Could you check a few things on this model? Use its own coordinates, in mm. Face numbers are marked on the shaded views. A direction names the side the tool comes from. Round coordinates to 2 decimals unless told otherwise and drop trailing zeros. Loops run counter-clockwise (first coordinate to the right, second up) from the corner with the lowest first, then second, coordinate; pieces in that order, holes last. Notation, with made-up numbers: (78, 12.5) -> (129, 12.5) arc R22 cw to (129, 36.5) -> close; hole circle Ø6 at (71.25, -0.5). An arc over 180 degrees is marked (long way). One line per item, written item: value.
Autodesk Inventor part; units mm, degrees
ref_plane "YZ Plane" through (0, 0, 0) normal (1, 0, 0) x (0, 1, 0)
ref_plane "XZ Plane" through (0, 0, 0) normal (0, 1, 0) x (-1, 0, 0)
ref_plane "XY Plane" through (0, 0, 0) normal (0, 0, 1) x (1, 0, 0)
sketch "Sketch1" plane through (0, 0, 0) normal (0, 0, 1) x (1, 0, 0)
  circle A0 centre (0, 0) radius 9.5
  arc A1 (2, 11.5) -> (-2, 11.5) centre (0, 11.5) ccw
  line L0 (-2, 11.5) -> (-2, 9.2871)
  line L1 (2, 11.5) -> (2, 9.2871)
  line L2 (11.5, -2) -> (9.2871, -2)
  arc A2 (11.5, -2) -> (11.5, 2) centre (11.5, 0) ccw
  line L3 (11.5, 2) -> (9.2871, 2)
  line L4 (-2, -11.5) -> (-2, -9.2871)
  arc A3 (-2, -11.5) -> (2, -11.5) centre (0, -11.5) ccw
  line L5 (2, -11.5) -> (2, -9.2871)
  line L6 (-11.5, 2) -> (-9.2871, 2)
  arc A4 (-11.5, 2) -> (-11.5, -2) centre (-11.5, 0) ccw
  line L7 (-11.5, -2) -> (-9.2871, -2)
  line L8 (0, 0) -> (6.7175, 6.7175) construction
  line L9 (0, 0) -> (9.5, 0) construction
  line L10 (5.7012, 8.8174) -> (4.9765, 8.0923)
  line L11 (8.8174, 5.7012) -> (8.0925, 4.9761)
  arc A5 (8.8174, 5.7012) -> (5.7012, 8.8174) centre (0, 0) ccw
  arc A6 (-10.3078, 2) -> (-10.3696, 1.6499) centre (0, 0) ccw
  arc A7 (-10.3696, -1.6499) -> (-10.3078, -2) centre (0, 0) ccw
  arc A8 (2, 10.3078) -> (1.6499, 10.3696) centre (0, 0) ccw
  arc A9 (-1.6499, 10.3696) -> (-2, 10.3078) centre (0, 0) ccw
  arc A10 (10.3078, -2) -> (10.5, 0) centre (0, 0) ccw
  arc A11 (10.3696, 1.6499) -> (10.3078, 2) centre (0, 0) ccw
  arc A12 (10.3078, -2) -> (10.3078, 2) centre (0, 0) ccw construction
  arc A13 (-2, -10.3078) -> (-1.6499, -10.3696) centre (0, 0) ccw
  arc A14 (1.6499, -10.3696) -> (2, -10.3078) centre (0, 0) ccw
  arc A15 (-2, -10.3078) -> (-1.6499, -10.3696) centre (0, 0) ccw construction
  arc A16 (1.6499, -10.3696) -> (2, -10.3078) centre (0, 0) ccw construction
  line L12 (-8.8174, -5.7012) -> (-8.0925, -4.9761)
  arc A17 (-8.8174, -5.7012) -> (-5.7012, -8.8174) centre (0, 0) ccw
  line L13 (-5.7012, -8.8174) -> (-4.9765, -8.0923)
  line L14 (7.4246, 7.4246) -> (0, 0) construction
  point P0 (-4.9765, -8.0923)
  dimension "d0" = 19
  dimension "d1" = 4
  dimension "d4" = 360
  dimension "d7" = 45
  dimension "d9" = 10.5
  dimension "d12" = 360
extrude "Extrusion1" add sketch "Sketch1" along normal blind 20 contours A0
extrude "Extrusion2" add sketch "Sketch1" along normal blind 7.5 contours A0 L3 A2 L2 | L5 A3 L4 A0 | A0 L0 A1 L1 | A0 L7 A4 L6
extrude "Extrusion3" add sketch "Sketch1" along normal blind 3 contours A0 L10 A5 L11 | L13 A17 L12 A0
sketch "Sketch2" plane through (0, 0, 20) normal (0, 0, 1) x (1, 0, 0)
  circle A0 centre (0, 0) radius 6.65
  dimension "d20" = 13.3
extrude "Extrusion4" add sketch "Sketch2" along normal blind 2
sketch "Sketch3" plane through (0, 0, 22) normal (0, 0, 1) x (1, 0, 0)
  circle A0 centre (0, 0) radius 2
  dimension "d23" = 4
extrude "Extrusion5" add sketch "Sketch3" along normal blind 8
properties part number "Solenoid Valve"
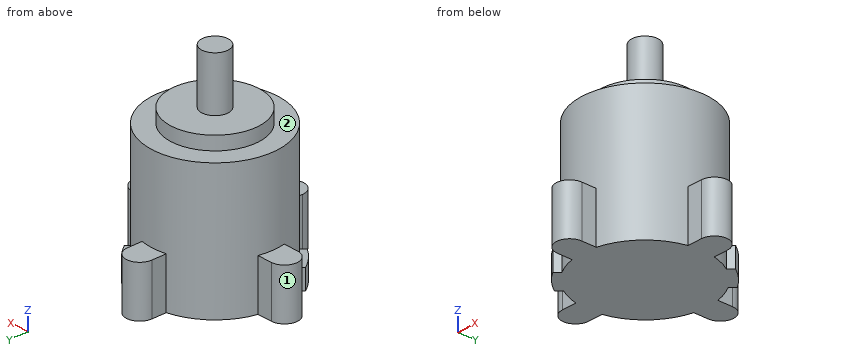
(1) If we section it at D-D, the plane y = -4: Please give me the cut outline in (x, z), then the cut area to 3 significant figures.
Recorded:
outline: (-8.62, 0) -> (8.62, 0) -> (8.62, 20) -> (5.31, 20) -> (5.31, 22) -> (-5.31, 22) -> (-5.31, 20) -> (-8.62, 20) -> close
area: 366 mm²
(2) If I drill on L1, parallel to Z at x = -5.25, y = 6.75; L2, parallel to X at y = 10.5, z = 4.75, over which ranges is the centre line in solid material (lowest first)?
Recorded:
L1: 0 to 20
L2: -2 to 2
(3) For the marked faces 1 and 2, which set-ups out of +Z, -Z, +X, -X, +Y, -Y let a thin tool reach every point of the face, with its end or its side?
Recorded:
face 1: +Z, -Z, -X
face 2: +Z
(4) If we section it at C-C, the plane z = 8.5: Please give me the cut outline in (x, y).
Recorded:
outline: circle Ø19 at (0, 0)
(5) If we section it at A-A, the plane x = 0: Please give me the cut outline in (y, z).
Recorded:
outline: (-13.5, 0) -> (13.5, 0) -> (13.5, 7.5) -> (9.5, 7.5) -> (9.5, 20) -> (6.65, 20) -> (6.65, 22) -> (2, 22) -> (2, 30) -> (-2, 30) -> (-2, 22) -> (-6.65, 22) -> (-6.65, 20) -> (-9.5, 20) -> (-9.5, 7.5) -> (-13.5, 7.5) -> close
(6) I'm going to push flat-ended pins straight in: pin 1 Ø1.5 at (x, y) = (5, -1) entering from +Z; pin 2 Ø0.7 at (x, z) = (-10.5, 3) entering from +Y; pin 3 Ø1.5 at (x, z) = (6, 14.5) entering from -Y. Where does each tip first touch, or does it pass through?
Recorded:
pin 1: z = 22
pin 2: y = 2
pin 3: y = -7.92
